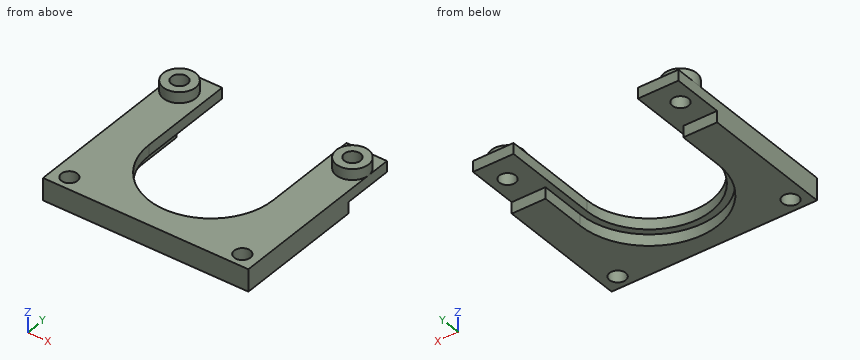
from build123d import *

# Parameters (mm, degrees)
SKETCH_1_R          = 1.5
EXTRUDE_1_DEPTH     = 4.1
EXTRUDE_START       = -2
EXTRUDE_2_DEPTH     = 2
SKETCH_3_W          = 78.409677764
SKETCH_3_H          = 10
CUT_EXTRUDE_1_DEPTH = 2.1
SKETCH_4_W          = 7.5
SKETCH_4_H          = 2
EXTRUDE_3_DEPTH     = 2
SKETCH_5_R          = 3
SKETCH_5_R_2        = 1.5
EXTRUDE_4_DEPTH     = 2


with BuildPart() as part:
    # 草图1 → 凸台-拉伸1 (new body)
    with BuildSketch(Plane.XY):
        with BuildLine():
            Line((-12.75, 0), (-12.75, 16))
            Line((-12.75, 16), (-19, 16))
            Line((-19, 16), (-19, -16))
            Line((-19, -16), (19, -16))
            Line((19, -16), (19, 16))
            Line((19, 16), (12.75, 16))
            Line((12.75, 16), (12.75, 0))
            ThreePointArc((12.75, 0), (0, -12.75), (-12.75, 0))
        make_face()
        with Locations((-16, 13.5)):
            Circle(SKETCH_1_R, mode=Mode.SUBTRACT)
        with Locations((16, 13.5)):
            Circle(SKETCH_1_R, mode=Mode.SUBTRACT)
        with Locations(Location((16, -13.5, 0), (0, 0, 180))):
            Circle(SKETCH_1_R, mode=Mode.SUBTRACT)
        with Locations(Location((-16, -13.5, 0), (0, 0, 180))):
            Circle(SKETCH_1_R, mode=Mode.SUBTRACT)
    extrude(amount=EXTRUDE_1_DEPTH)

    # 草图2 → 凸台-拉伸2 (add)
    with BuildSketch(Plane.XY.offset(4.1).offset(EXTRUDE_START)):
        with BuildLine():
            Line((-12.75, 0), (-12.75, 16))
            Line((-12.75, 16), (-11.5, 16))
            Line((-11.5, 16), (-11.5, 0))
            ThreePointArc((-11.5, 0), (0, -11.5), (11.5, 0))
            Line((11.5, 0), (11.5, 16))
            Line((11.5, 16), (12.75, 16))
            Line((12.75, 16), (12.75, 0))
            ThreePointArc((12.75, 0), (0, -12.75), (-12.75, 0))
        make_face()
    extrude(amount=EXTRUDE_2_DEPTH)

    # 草图3 → 切除-拉伸1 (cut)
    with BuildSketch(Plane(origin=(0, 0, 0), x_dir=(-1, 0, 0), z_dir=(0, 0, -1))):
        with Locations((16, 13.5)):
            Rectangle(SKETCH_3_W, SKETCH_3_H)
    extrude(amount=-CUT_EXTRUDE_1_DEPTH, mode=Mode.SUBTRACT)

    # 草图4 → 凸台-拉伸3 (add)
    with BuildSketch(Plane.XY.offset(4.1)):
        with Locations((-15.25, 17)):
            Rectangle(SKETCH_4_W, SKETCH_4_H)
        with Locations((15.25, 17)):
            Rectangle(SKETCH_4_W, SKETCH_4_H)
    extrude(amount=-EXTRUDE_3_DEPTH)

    # 草图5 → 凸台-拉伸4 (add)
    # profile 1 of 2: a face of its own
    with BuildSketch(Plane.XY.offset(4.1)):
        with Locations(Location((-16, 13.5, 0), (0, 0, 180))):
            Circle(SKETCH_5_R)
        with Locations((-16, 13.5)):
            Circle(SKETCH_5_R_2, mode=Mode.SUBTRACT)
    # profile 2 of 2: a face of its own
    with BuildSketch(Plane.XY.offset(4.1)):
        with Locations((16, 13.5)):
            Circle(SKETCH_5_R)
        with Locations((16, 13.5)):
            Circle(SKETCH_5_R_2, mode=Mode.SUBTRACT)
    extrude(amount=EXTRUDE_4_DEPTH)


solid = part.part
Geometry: final body of the model. Coordinates: model frame, mm. Coordinates: 2 decimals unless noted, no trailing zeros. Loops run counter-clockwise (first coordinate to the right, second up) from the corner with the lowest first, then second, coordinate; pieces in that order, holes last. Notation, with made-up numbers: M 35,5.25 L 46,5.25 A28 cw 46,30.25 Z; hole C 6,8 d8. An arc over 180 degrees is marked long. One line per item, written item: value. Start each with the question number.
1) Pin query (flat end, axial travel): P1, Ø5, axis at x = 16, y = 13.5, coming from the -Z side; P2, Ø2.5, axis at x = -16, y = 13.5, coming from the +Z side; P3, Ø2.5, axis at x = -16.5, z = 0.5, coming from the +Y side; P4, Ø17, axis at x = -1, y = -4.5, coming from the +Z side. Return the tip coordinate at first contact, or that it passes through.
2) Cut plane D-D (y = 3). Return loops of the section in (x, z), then the cut area to 4 significant figures.
3) Material intervals for L1, parallel to X at y = 13.5, z = 3.1; L2, parallel to X at y = -13.5, z = 1.9; L3, parallel to Y at x = 16, z = 2.95, sorted ascending. Write a range as from..to.
4) Cut plane B-B (z = 5.5). Return loops of the section in (x, y), then the cut area to 3 significant figures.
5) Cut plane A-A (y = -13.5). Return loops of the section in (x, z).
6) Cut plane C-C (x = -16). Return loops of the section in (y, z).
Evaluation:
1. P1: z = 2.1
1. P2: through
1. P3: y = 8.5
1. P4: z = 4.1
2. outline: M -19,0 L -12.75,0 L -12.75,2.1 L -11.5,2.1 L -11.5,4.1 L -19,4.1 Z; M 11.5,2.1 L 12.75,2.1 L 12.75,0 L 19,0 L 19,4.1 L 11.5,4.1 Z
2. area: 56.25 mm^2
3. L1: -19..-17.5, -14.5..-11.5, 11.5..14.5, 17.5..19
3. L2: -19..-17.5, -14.5..14.5, 17.5..19
3. L3: -16..-15, -12..12, 15..18
4. outline: C -16,13.5 d6; C 16,13.5 d6; hole C -16,13.5 d3; hole C 16,13.5 d3
4. area: 42.4 mm^2
5. outline: M -19,0 L -17.5,0 L -17.5,4.1 L -19,4.1 Z; M -14.5,0 L 14.5,0 L 14.5,4.1 L -14.5,4.1 Z; M 17.5,0 L 19,0 L 19,4.1 L 17.5,4.1 Z
6. outline: M -16,0 L -15,0 L -15,4.1 L -16,4.1 Z; M -12,0 L 8.5,0 L 8.5,2.1 L 12,2.1 L 12,6.1 L 10.5,6.1 L 10.5,4.1 L -12,4.1 Z; M 15,2.1 L 18,2.1 L 18,4.1 L 16.5,4.1 L 16.5,6.1 L 15,6.1 Z
